```python
from build123d import *

# Parameters (mm, degrees)
SKETCH1_R           = 6.223
BOSS_EXTRUDE1_DEPTH = 33.02
SKETCH2_R           = 12.446
BOSS_EXTRUDE2_DEPTH = 33.02
SKETCH3_W           = 3.302
SKETCH3_H           = 3.302
BOSS_EXTRUDE3_DEPTH = 12.7
SKETCH4_R           = 11.938
CUT_EXTRUDE1_DEPTH  = 1.1684


with BuildPart() as part:
    # Sketch1 → Boss-Extrude1 (new body)
    with BuildSketch(Plane.XY):
        Circle(SKETCH1_R)
    extrude(amount=BOSS_EXTRUDE1_DEPTH)

    # Sketch2 → Boss-Extrude2 (add)
    with BuildSketch(Plane.XY.offset(33.02)):
        Circle(SKETCH2_R)
    extrude(amount=BOSS_EXTRUDE2_DEPTH)

    # Sketch3 → Boss-Extrude3 (add)
    with BuildSketch(Plane(origin=(0, 0, 0), x_dir=(-1, 0, 0), z_dir=(0, 0, -1))):
        with Locations((0, 5.999994)):
            Rectangle(SKETCH3_W, SKETCH3_H)
    extrude(amount=-BOSS_EXTRUDE3_DEPTH)

    # Sketch4 → Cut-Extrude1 (cut)
    with BuildSketch(Plane.XY.offset(35.56)):
        Polygon((-17.203352379, 15.291868781), (-17.203352379, -16.384145123), (20.97667065, -17.277825766), (19.785096459, 16.68203867), align=None)
        Circle(SKETCH4_R, mode=Mode.SUBTRACT)
    extrude(amount=-CUT_EXTRUDE1_DEPTH, mode=Mode.SUBTRACT)


solid = part.part
```
Read the model definition and answer for the solid it produces. Units are mm, in the model's axes. A direction names the side the tool comes from. Give positions to 0.01 mm unless a question says otherwise; leave off trailing zeros. Order: outer loops, then holes, each group sorted by start corner. A loop starts at its lowest first (then second) coordinate and runs counter-clockwise, first axis right, second up. Notation, with made-up numbers: (1.5, 54) -> (22.5, 54) arc R13 cw to (22.5, 72) -> close; hole circle Ø7 at (13.25, -10). An arc over 180 degrees is marked (long way). One line per item, written item: value. Start each with the question number.
(1) Flat-ended cylindrical pins translate along their axes: P1, Ø5, axis at y = 5, z = 52.5, coming from the +X side; P2, Ø0.8, axis at y = 6.5, z = 4, coming from the -X side; P3, Ø12, axis at y = -7, z = 51.5, coming from the +X side; P4, Ø12, axis at x = 4.5, z = 30, coming from the +Y side. Find the tip coordinate at first contact, or state that the pin passes through.
(2) The part is cut by section B-B (x = 0). Determine the outline of the cut face in (y, z), and give its area (3 significant figures).
(3) A tool of negligible diameter and unlimited length cuts with its end or side. For faces 4 (the cylindrical face through (-2.588, -11.654, 34.984)), 5 (the flat face through (-1.651, 7, 6)), 6 (the flat face through (0, 7.651, 6)), from which of +Z, -Z, +X, -X, +Y, -Y can it reach the whole face along a straight path? Write none if from no direction.
(4) The part is cut by section A-A (y = 7). Determine the outline of the cut face in (x, z).
(5) For a pull along Z with two mould halves and no side action, classify faces 1 (the flat face through (1.651, 7, 6)), 2 (the flat face through (0, 7, 12.7)), 3 (the flat face through (0, 1, 0)) as released by +Z, released by -Z, zero draft, split by the parting line, or undercut.
(6) The part is cut by section D-D (y = -7). Determine the outline of the cut face in (x, z), and give its area (3 significant figures).
(7) The part is cut by section C-C (z = 49.5). Determine the outline of the cut face in (x, y), and give its area (3 significant figures).
(8) Straight lines are drawn through the part: L1, parallel to Z at x = 5.5, y = 8.5; L2, parallel to Y at x = 3.5, z = 42.5; L3, parallel to X at y = -2, z = 63. For each, find the intervals that lie inside material, in ascending order.
Taken from the geometry:
1. P1: x = 12.19
1. P2: x = -1.65
1. P3: x = 12.41
1. P4: y = 12.45
2. outline: (-12.45, 33.02) -> (-6.22, 33.02) -> (-6.22, 0) -> (7.65, 0) -> (7.65, 12.7) -> (6.22, 12.7) -> (6.22, 33.02) -> (12.45, 33.02) -> (12.45, 34.39) -> (11.94, 34.39) -> (11.94, 35.56) -> (12.45, 35.56) -> (12.45, 66.04) -> (-12.45, 66.04) -> (-12.45, 35.56) -> (-11.94, 35.56) -> (-11.94, 34.39) -> (-12.45, 34.39) -> close
2. area: 1,250 mm^2
3. face 4: none
3. face 5: -Z, -X, +Y
3. face 6: -Z, +X, -X, +Y
4. outline: (-10.29, 33.02) -> (10.29, 33.02) -> (10.29, 34.39) -> (9.67, 34.39) -> (9.67, 35.56) -> (10.29, 35.56) -> (10.29, 66.04) -> (-10.29, 66.04) -> (-10.29, 35.56) -> (-9.67, 35.56) -> (-9.67, 34.39) -> (-10.29, 34.39) -> close; (-1.65, 0) -> (1.65, 0) -> (1.65, 12.7) -> (-1.65, 12.7) -> close
5. face 1: zero draft
5. face 2: undercut
5. face 3: released by -Z
6. outline: (-10.29, 33.02) -> (10.29, 33.02) -> (10.29, 34.39) -> (9.67, 34.39) -> (9.67, 35.56) -> (10.29, 35.56) -> (10.29, 66.04) -> (-10.29, 66.04) -> (-10.29, 35.56) -> (-9.67, 35.56) -> (-9.67, 34.39) -> (-10.29, 34.39) -> close
6. area: 678 mm^2
7. outline: circle Ø24.89 at (0, 0)
7. area: 487 mm^2
8. L1: 33.02 to 66.04
8. L2: -11.94 to 11.94
8. L3: -12.28 to 12.28
